Design review of the part built by this model. Coordinates are the model's own, in mm. A direction names the side the tool comes from. Coordinates: 2 decimals unless noted, no trailing zeros. Write each loop counter-clockwise with the first axis right and the second up, starting at its lowest first coordinate (ties: lowest second). Pieces come first, ordered by that corner, then holes. Notation, with made-up numbers: (2.5, 75) -> (18.5, 75) arc R30 cw to (18.5, 97) -> close; hole circle Ø6 at (-16, 1). An arc over 180 degrees is marked (long way). Answer in a Markdown table with one row per item. Add a question column.
Item 1: For faces 1 (the face through (25.35, -19.488, 61.257)), 2 (the face through (25.361, 50.133, 1.432)), 3 (the face through (20.4, 47.8, 14.7)), list the 3-axis set-ups (+Z, -Z, +X, -X, +Y, -Y) from which the entire face can be reached by the end or side of a thin tool; tool diameter is ignored.
Item 2: Take a section at B-B, the plane z = 86.5. Write out the cut boundary in (x, y), and give its area (3 significant figures).
Item 3: Draft analysis for pull direction Y (two halves, no side actions). For faces 4 (the face through (25, -17, 69.5)), 5 (the face through (11.633, 64.095, 2.641)), 6 (the face through (25.35, 24.601, 66.263)), state which applies: released by +Y, released by -Y, zero draft, split by the parting line, or undercut.
Item 4: Take a section at D-D, the plane x = 28.5. Give the number of separate pieces and of enclosed holes in the cut face, and give its area (3 significant figures).
Item 5: Take a section at C-C, the plane y = -68. Write out the cut boundary in (x, z), and give its area (3 significant figures).
Item 6: Clearance check with flat-ended pins moving along their axes: P1, Ø10.5, axis at x = 12.5, y = -68, coming from the -Z side; P2, Ø9.5, axis at x = 19.5, y = -71.5, coming from the +Z side; P3, Ø5, axis at x = 45, y = -9, coming from the +Z side; P4, Ø7, axis at x = 37.5, y = -68, coming from the +Z side. State where each tip first meets the part, or that it passes through.
Item 7: To check wall thickness, follow line 1 (X direction, y = 0, z = 65.75); line 2 (Y direction, x = 37, z = 3); line 3 (Y direction, x = 4.5, z = 68). State the ranges of each line that lie inside material, in increasing order.
Item 8: Take a section at A-A, the plane y = 0. Write out the cut boundary in (x, z).
Solid Edge part; units mm, degrees
sketch "Sketch1" plane through (0, 0, 0) normal (1, 0, 0) x (0, 1, 0)
  line L0 (-50, 0) -> (-20, 62)
  line L1 (-20, 62) -> (20, 62)
  line L2 (50, 0) -> (20, 62)
  line L3 (50, 0) -> (79.8022, 0)
  line L4 (79.8022, 0) -> (79.8022, 5)
  line L5 (79.8022, 5) -> (57.8022, 5)
  line L6 (25, 67) -> (57.8022, 5)
  line L7 (-25, 67) -> (25, 67)
  line L8 (-55, 5) -> (-25, 67)
  line L9 (-77, 5) -> (-55, 5)
  line L10 (-77, 0) -> (-77, 5)
  line L11 (-77, 0) -> (-50, 0)
  dimension "D1" = 20
  dimension "D2" = 79.8022
  dimension "D3" = 79.8022
  dimension "D4" = 77
  dimension "D5" = 25
  dimension "D6" = 77
extrude "Protrusion1" add sketch "Sketch1" along normal blind 50
sketch "Sketch2" plane through (25, 0, 67) normal (0, 0, 1) x (1, 0, 0)
  line L0 (-25, 20) -> (25, 20)
  line L1 (25, 20) -> (25, 15)
  line L2 (25, 15) -> (-25, 15)
  line L3 (-25, 15) -> (-25, 20)
  line L4 (-25, -20) -> (25, -20)
  line L5 (25, -20) -> (25, -15)
  line L6 (25, -15) -> (-25, -15)
  line L7 (-25, -15) -> (-25, -20)
  dimension "D1" = 25
extrude "ExtrudedProtrusion_2" add sketch "Sketch2" along normal blind 2.5
sketch "Sketch3" plane through (25, -66, 5) normal (0, 0, 1) x (1, 0, 0)
  circle A0 centre (-12.5, -2) radius 4
  circle A1 centre (12.5, -2) radius 4
  dimension "D1" = 12.5
extrude "Cutout1" cut sketch "Sketch3" against normal up to next
mirror "Mirror1" about plane through (0, 0, 0) normal (0, -1, 0) of "Cutout1"
sketch "Sketch4" plane through (25, 0, 67) normal (0, 0, 1) x (0, 1, 0)
  circle A0 centre (0, -17.5) radius 2.5
  circle A1 centre (0, 15) radius 2.5
extrude "Cutout2" cut sketch "Sketch4" against normal up to next
sketch "Sketch5" plane through (0, 0, 0) normal (0, 1, 0) x (-1, 0, 0)
  line L0 (0, 0) -> (-66.0658, 1.6838)
  line L1 (-66.0658, 1.6838) -> (-66.0658, 0)
  line L2 (-66.0658, 0) -> (0, 0)
extrude "ExtrudedCutout_3" cut sketch "Sketch5" along normal mid plane 208
fillet "Round_1" radius 5 8 edges at (25, 25, 67) (25, 49.6917, 0.6372) (25, 57.8022, 5) (25, -25, 67) (25, -20, 62) (25, -49.6917, 0.6372) (25, -55, 5) (25, 20, 62)
sketch "Sketch6" plane through (25, 41.4011, 36) normal (0, 0.8839, 0.4677) x (-1, 0, 0)
  circle A0 centre (0, 17.06) radius 10
  circle A1 centre (0, -12.94) radius 10
extrude "Cutout3" cut sketch "Sketch6" against normal up to next
mirror "Mirror2" about plane through (0, 0, 0) normal (0, -1, 0) of "Cutout3"
sketch "Sketch7" plane through (25, 0, 67) normal (0, 0, 1) x (0, 1, 0)
  circle A0 centre (0, -9.19) radius 2.5
extrude "Protrusion2" add sketch "Sketch7" along normal blind 25
properties material "Stainless steel"
Answers:
| question | item | result |
|---|---|---|
| 1 | face 1 | -Z, +X, -X |
| 1 | face 2 | -Z, +X |
| 1 | face 3 | none |
| 2 | outline | circle Ø5 at (34.19, 0) |
| 2 | area | 19.6 mm^2 |
| 3 | face 4 | zero draft |
| 3 | face 5 | undercut |
| 3 | face 6 | released by +Y |
| 4 | separate pieces | 5 |
| 4 | enclosed holes | 0 |
| 4 | area | 929 mm^2 |
| 5 | outline | (0, 0) -> (8.5, 0.22) -> (8.5, 5) -> (0, 5) -> close; (16.5, 0.42) -> (33.5, 0.85) -> (33.5, 5) -> (16.5, 5) -> close; (41.5, 1.06) -> (50, 1.27) -> (50, 5) -> (41.5, 5) -> close |
| 5 | area | 148 mm^2 |
| 6 | P1 | stops at z = 0.18 |
| 6 | P2 | stops at z = 5 |
| 6 | P3 | stops at z = 67 |
| 6 | P4 | passes through |
| 7 | line 1 | x = 0 to 7.5, 12.5 to 40, 45 to 50 |
| 7 | line 2 | y = -77 to -71.97, -64.03 to -48.64, 48.64 to 64.03, 71.97 to 79.8 |
| 7 | line 3 | y = -20 to -15, 15 to 20 |
| 8 | outline | (0, 62) -> (7.5, 62) -> (7.5, 67) -> (0, 67) -> close; (12.5, 62) -> (40, 62) -> (40, 67) -> (36.69, 67) -> (36.69, 92) -> (31.69, 92) -> (31.69, 67) -> (12.5, 67) -> close; (45, 62) -> (50, 62) -> (50, 67) -> (45, 67) -> close |
